```python
from build123d import *

# Parameters (mm, degrees)
F0_W     = 100
F0_H     = 100
F1_DEPTH = 50
F2_R     = 36.4914708522
F3_DEPTH = 100.001


with BuildPart() as f1:
    # F0 (on Front) → F1 (new body, symmetric)
    with BuildSketch(Plane.XZ):
        Rectangle(F0_W, F0_H)
    extrude(amount=F1_DEPTH, both=True)

    # F2 (on face) → F3 (cut, through all)
    with BuildSketch(Plane.XY.offset(50)):
        Circle(F2_R)
    extrude(amount=-F3_DEPTH, mode=Mode.SUBTRACT)


solid = f1.part
```
Here's how the part is built. I have some questions about the finished solid (model axes, mm). Give positions to 0.01 mm unless a question says otherwise; leave off trailing zeros. Loops run counter-clockwise (first coordinate to the right, second up) from the corner with the lowest first, then second, coordinate; pieces in that order, holes last. Notation, with made-up numbers: M -1.75,-0.75 L 54.25,-0.75 A16 cw 54.25,5.25 Z; hole C -40,25 d1. An arc over 180 degrees is marked long. Put each result on its own line as item: value. Start each with the question number.
(1) If we mould it in two halves opening along X, with no side actions, what happens to faces 1 (the flat face through (50, -1, -1)), 2 (the cylindrical face through (-28.96, -22.2, 0.7)), 3 (the flat face through (-34, -23, 50))? For each: +X half, -X half, draft (parallel to the pull), parting line (faces both ways), or undercut.
(2) I need wall thicknesses on line 1 along Y through (x, z) = (0, 15.5); line 2 along X through (y, z) = (-15, -18.5); line 3 along Y through (x, z) = (-14, 29). Which ranges of each line are inside material? Lowest first, please. Write a range as [from, to].
(3) I want a section at A-A on y = 0. Please give me the cut outline in (x, z).
(4) I want a section at C-C on z = -40. Please give me the cut outline in (x, y), then the cut area to 3 significant figures.
Answer block:
1. face 1: +X half
1. face 2: undercut
1. face 3: draft
2. line 1: [-50, -36.49], [36.49, 50]
2. line 2: [-50, -33.27], [33.27, 50]
2. line 3: [-50, -33.7], [33.7, 50]
3. outline: M -50,-50 L -36.49,-50 L -36.49,50 L -50,50 Z; M 36.49,-50 L 50,-50 L 50,50 L 36.49,50 Z
4. outline: M -50,-50 L 50,-50 L 50,50 L -50,50 Z; hole C 0,0 d72.98
4. area: 5,820 mm^2
